Verification items for the finished model (mm, model axes). Face numbers are marked on the shaded views. A direction names the side the tool comes from. Coordinates: 2 decimals unless noted, no trailing zeros. Write each loop counter-clockwise with the first axis right and the second up, starting at its lowest first coordinate (ties: lowest second). Pieces come first, ordered by that corner, then holes. Notation, with made-up numbers: (59, 51.5) -> (63, 51.5) arc R16 ccw to (63, 70.5) -> close; hole circle Ø8 at (-22, -14.75). An arc over 180 degrees is marked (long way). Answer in a Markdown table with one row per item.
```python
from build123d import *

# Parameters (mm, degrees)
F0_W     = 101.6
F0_H     = 76.2
F1_DEPTH = 50.8
F2_W     = 76.2
F2_H     = 50.8
F3_DEPTH = 50.8
F4_W     = 25.4
F4_H     = 25.4
F6_R     = 12.7
F7_DEPTH = 101.6
F9_DEPTH = 101.6


with BuildPart() as f1:
    # F0 (on Front) → F1 (new body)
    with BuildSketch(Plane.XZ):
        with Locations((3.755716607, -12.4916662514)):
            Rectangle(F0_W, F0_H)
    extrude(amount=F1_DEPTH)

    # F2 (on face) → F3 (cut)
    with BuildSketch(Plane.XY.offset(25.6083337486)):
        with Locations((16.455716607, -25.4)):
            Rectangle(F2_W, F2_H)
    extrude(amount=-F3_DEPTH, mode=Mode.SUBTRACT)

    # F4 (on face) → F5 (revolve)
    with BuildSketch(Plane.YZ.offset(54.555716607)):
        with Locations((-12.7, -37.8916662514)):
            Rectangle(F4_W, F4_H)
    revolve(axis=Axis((54.555716607, -25.4, -37.8916662514), (0, 0, -1)))

    # F6 (on face) → F7 (cut)
    with BuildSketch(Plane.XY.offset(-25.1916662514)):
        with Locations((0, -25.4)):
            Circle(F6_R)
        with Locations((48.030372709, -25.4)):
            Circle(F6_R)
    extrude(amount=-F7_DEPTH, mode=Mode.SUBTRACT)

    # F8 (on face) → F9 (cut)
    with BuildSketch(Plane.YZ.offset(-21.644283393)):
        with BuildLine():
            Line((-3.748458612, 25.6083337486), (-48.2540987432, 25.6083337486))
            ThreePointArc((-48.2540987432, 25.6083337486), (-26.0012786776, -2.4853646692), (-3.748458612, 25.6083337486))
        make_face()
    extrude(amount=-F9_DEPTH, mode=Mode.SUBTRACT)


solid = f1.part
```
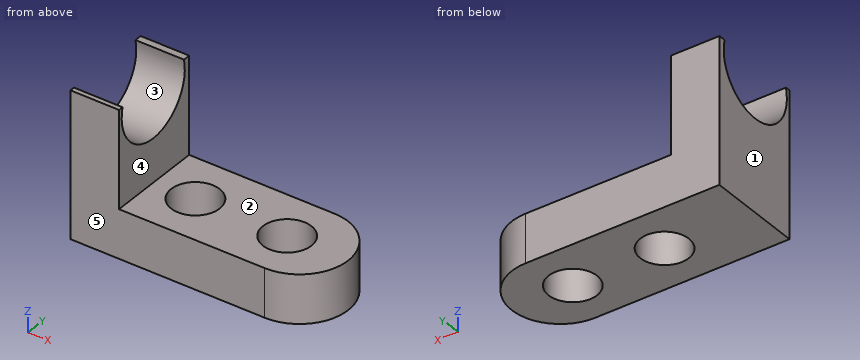
1. Sectioned sample at A-A, the plane x = 0. Record the cut outline in (y, z), and give its area (3 significant figures).
Findings below:
| item | result |
|---|---|
| outline | (-50.8, -50.59) -> (-38.1, -50.59) -> (-38.1, -25.19) -> (-50.8, -25.19) -> close; (-12.7, -50.59) -> (0, -50.59) -> (0, -25.19) -> (-12.7, -25.19) -> close |
| area | 645 mm² |
2. Sectioned sample at B-B, the plane y = -25.4. Record the cut outline in (x, z), and give its area (3 significant figures).
Findings below:
| item | result |
|---|---|
| outline | (-47.04, -50.59) -> (-12.7, -50.59) -> (-12.7, -25.19) -> (-21.64, -25.19) -> (-21.64, -2.48) -> (-47.04, -2.48) -> close; (12.7, -50.59) -> (35.33, -50.59) -> (35.33, -25.19) -> (12.7, -25.19) -> close; (60.73, -50.59) -> (79.96, -50.59) -> (79.96, -25.19) -> (60.73, -25.19) -> close |
| area | 2,510 mm² |
3. Go/stop test with flat-tipped pins: pin 1 (6 mm diameter, centred on x = -7.5, y = -37.5, fed in from +Z); pin 2 (1.5 mm diameter, centred on y = -34.5, z = -29, fed in from +X); pin 3 (5 mm diameter, centred on x = -24, y = -17.5, fed in from +Z). Record where each tip stops, or that it passes through.
Findings below:
| item | result |
|---|---|
| pin 1 | stops at z = -25.19 |
| pin 2 | stops at x = 78.54 |
| pin 3 | stops at z = 0.34 |
4. Sectioned sample at D-D, the plane x = -27.5. Record the cut outline in (y, z).
Findings below:
| item | result |
|---|---|
| outline | (-50.8, -50.59) -> (0, -50.59) -> (0, 25.61) -> (-3.75, 25.61) arc R22.86 cw (long way) to (-48.25, 25.61) -> (-50.8, 25.61) -> close |
5. Access from +Z, -Z, +X, -X, +Y, -Y to the whole of each face (thin tool, end or side, straight path). Record for the marked faces 4 and 5.
Findings below:
| item | result |
|---|---|
| face 4 | +Z, +X, +Y, -Y |
| face 5 | +Z, -Z, +X, -X, -Y |
6. Material ranges on probe 1 along X at (y, z) = (-25, -40); probe 2 along Y at (x, z) = (0, -39.75); probe 3 along X at (y, z) = (-20, -45), recorded low to high. Write a range as from..to.
Findings below:
| item | result |
|---|---|
| probe 1 | x = -47.04..-12.69, 12.69..35.34, 60.72..79.95 |
| probe 2 | y = -50.8..-38.1, -12.7..0 |
| probe 3 | x = -47.04..-11.49, 11.49..36.54, 59.53..79.38 |
7. Sectioned sample at C-C, the plane z = 9. Record the cut outline in (x, y), and give its area (3 significant figures).
Findings below:
| item | result |
|---|---|
| outline | (-47.04, -50.8) -> (-21.64, -50.8) -> (-21.64, -45.83) -> (-47.04, -45.83) -> close; (-47.04, -6.17) -> (-21.64, -6.17) -> (-21.64, 0) -> (-47.04, 0) -> close |
| area | 283 mm² |
8. Release check for a two-part mould opening along Z. For the marked faces 1, 2 and 3 record: released by +Z, released by -Z, zero draft, split by the parting line, or undercut.
Findings below:
| item | result |
|---|---|
| face 1 | zero draft |
| face 2 | released by +Z |
| face 3 | undercut |
